from build123d import *

# Parameters (mm, degrees)
SKETCH1_R               = 9.5
SKETCH1_R_2             = 6.5
BOSS_EXTRUDE1_DEPTH     = 13.5
CUT_EXTRUDE1_REACH      = 29.046
CUT_EXTRUDE1_END_RADIUS = 6.5
CUT_EXTRUDE1_START      = -8
SKETCH2_W               = 3
SKETCH2_H               = 5


with BuildPart() as part:
    # Sketch1 → Boss-Extrude1 (new, symmetric)
    with BuildSketch(Plane.XY):
        Circle(SKETCH1_R)
        Circle(SKETCH1_R_2, mode=Mode.SUBTRACT)
    extrude(amount=BOSS_EXTRUDE1_DEPTH, both=True)

    # Cut-Extrude1: up to this cylinder (the profile starts outside it)
    cut_extrude1_end = Plane(origin=(0, 0, 11), z_dir=(0, 0, -1)) * Cylinder(CUT_EXTRUDE1_END_RADIUS, 72.092, mode=Mode.PRIVATE)
    # Sketch2 → Cut-Extrude1 (cut, up to the surface)
    with BuildSketch(Plane(origin=(0, 0, 0), x_dir=(1, 0, 0), z_dir=(0, 1, 0)).offset(CUT_EXTRUDE1_START), mode=Mode.PRIVATE) as cut_extrude1_sk1:
        with Locations((0, -11)):
            Rectangle(SKETCH2_W, SKETCH2_H)
    cut_extrude1_tool1 = extrude(cut_extrude1_sk1.sketch, amount=CUT_EXTRUDE1_REACH, mode=Mode.PRIVATE) - cut_extrude1_end
    add(cut_extrude1_tool1.solids().sort_by_distance((0, -8, 11))[0], mode=Mode.SUBTRACT)


solid = part.part
Input: part model. Units: mm. Frame: model coordinates. A direction names the side the tool comes from. Coordinates: 2 decimals unless noted, no trailing zeros. Order: outer loops, then holes, each group sorted by start corner. A loop starts at its lowest first (then second) coordinate and runs counter-clockwise, first axis right, second up.
1. Ray query, line 1 along Y through (x, z) = (0, -2.25); line 2 along Y through (x, z) = (1, -10.75); line 3 along X through (y, z) = (-4.5, -4). Return the intervals inside material, ascending.
Checked values:
line 1: y = -9.5 to -6.5, 6.5 to 9.5
line 2: y = -9.45 to -6.42, 6.42 to 9.45
line 3: x = -8.37 to -4.69, 4.69 to 8.37
2. Contact query for flat-ended pins moving along their axis: P1, Ø0.8, axis at y = -7, z = 11.5, coming from the -X side; P2, Ø0.8, axis at x = 0, y = -7, coming from the +Z side; P3, Ø2, axis at y = 2, z = 5, coming from the -X side; P4, Ø1, axis at x = -4.5, y = 3, coming from the +Z side. Output: stop coordinate, or through.
Checked values:
P1: stops at x = -6.83
P2: stops at z = 8.5
P3: stops at x = -9.45
P4: passes through
3. Cut plane C-C, the plane z = -5.5. Return loops of the section in (x, y), plus the area to 3 significant figures.
Checked values:
outline: circle Ø19 at (0, 0); hole circle Ø13 at (0, 0)
area: 151 mm2
4. Cut plane B-B, the plane x = 0. Return loops of the section in (y, z).
Checked values:
outline: (-9.5, -13.5) - (-6.5, -13.5) - (-6.5, 8.5) - (-8, 8.5) - (-8, 13.5) - (-9.5, 13.5) - close; (6.5, -13.5) - (9.5, -13.5) - (9.5, 13.5) - (6.5, 13.5) - close
5. Cut plane A-A, the plane y = 0. Return loops of the section in (x, z), plus the area to 3 significant figures.
Checked values:
outline: (-9.5, -13.5) - (-6.5, -13.5) - (-6.5, 13.5) - (-9.5, 13.5) - close; (6.5, -13.5) - (9.5, -13.5) - (9.5, 13.5) - (6.5, 13.5) - close
area: 162 mm2
6. Access query for faces 1 (the flat face through (1.5, -7, 11)), 2 (the flat face through (4, -6, -13.5)). Directions: +Z, -Z, +X, -X, +Y, -Y. A direction counts if a zero-diameter tool reaches every point of the face in a straight line with its end or side. Return the directions, or none.
Checked values:
face 1: +Z
face 2: -Z, +X, -X, +Y, -Y
7. Cut plane D-D, the plane x = -5. Return loops of the section in (y, z).
Checked values:
outline: (-8.08, -13.5) - (-4.15, -13.5) - (-4.15, 13.5) - (-8.08, 13.5) - close; (4.15, -13.5) - (8.08, -13.5) - (8.08, 13.5) - (4.15, 13.5) - close
